The drawing under review shows one solid part. Ordinate dimensions are in mm from its lowest x, y, z. A direction names the side the tool comes from. Round coordinates to 2 decimals unless told otherwise and drop trailing zeros. Write each loop counter-clockwise with the first axis right and the second up, starting at its lowest first coordinate (ties: lowest second). Pieces come first, ordered by that corner, then holes. Notation, with made-up numbers: M 16,-37.5 L 42,-37.5 A23 cw 42,-21.5 Z; hole C 15.25,-2 d2. An arc over 180 degrees is marked long. One line per item, written item: value. Start each with the question number.
1) Take a section at D-D, the plane z = 0.7. Write out the cut boundary in (x, y), and give its area (3 significant figures).
2) For P1, Ø2.5, axis at x = 3.5, y = 4, coming from the +Z side; P2, Ø1, axis at y = 5.5, z = 0.5, coming from the -X side; P3, Ø1, axis at y = 7, z = 1, coming from the -X side, all flat-tipped, find the tip position at first contact; note any pin that passes through.
3) Take a section at B-B, the plane z = 1.85. Write out the cut boundary in (x, y), and give its area (3 significant figures).
4) Wall thickness on probe 1 along Z at (x, y) = (4.5, 4); probe 2 along Y at (x, z) = (4.5, 1.8); probe 3 along X at (y, z) = (1.25, 1.1): over which ranges is each line inside the solid? List them lowest first.
5) Tool access review of the marked faces 1 and 2: name each direction out of +Z, -Z, +X, -X, +Y, -Y from which nothing blocks a thin tool from reaching the whole face with its end or side.
6) Mouldability with a two-part tool opening along Y and no side actions: class the marked faces 3, 4 and 5 as +Y half, -Y half, draft (parallel to the pull), parting line (faces both ways), or undercut.
7) Take a section at A-A, the plane y = 4. Write out the cut boundary in (x, z), and give its area (3 significant figures).
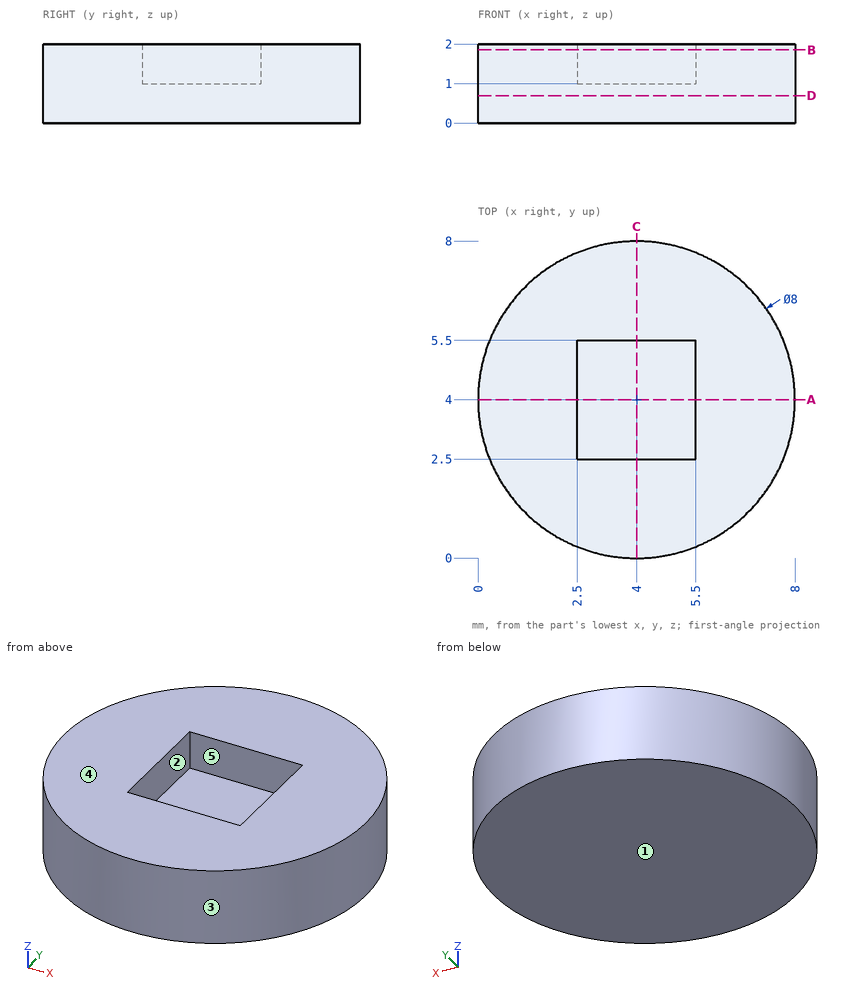
Checked values:
1. outline: C 4,4 d8
1. area: 50.3 mm2
2. P1: stops at z = 2
2. P2: stops at x = 0.13
2. P3: stops at x = 0.88
3. outline: C 4,4 d8; hole M 2.5,2.5 L 5.5,2.5 L 5.5,5.5 L 2.5,5.5 Z
3. area: 41.3 mm2
4. probe 1: z = 0 to 1
4. probe 2: y = 0.03 to 2.5, 5.5 to 7.97
4. probe 3: x = 1.1 to 6.9
5. face 1: -Z, +X, -X, +Y, -Y
5. face 2: +Z
6. face 3: parting line
6. face 4: draft
6. face 5: undercut
7. outline: M 0,0 L 8,0 L 8,2 L 5.5,2 L 5.5,1 L 2.5,1 L 2.5,2 L 0,2 Z
7. area: 13.0 mm2
